```python
from build123d import *

# Parameters (mm, degrees)
F0_R     = 99.8962025771
F1_DEPTH = 50
F2_R     = 7.3881969702
F3_DEPTH = 50.001
F4_DEPTH = 50
F5_DEPTH = 20


with BuildPart() as f1:
    # F0 (on Front) → F1 (new body)
    with BuildSketch(Plane.XZ):
        Circle(F0_R)
    extrude(amount=F1_DEPTH)

    # F2 (on face) → F3 (cut, through all)
    with BuildSketch(Plane.XZ.offset(50)):
        Circle(F2_R)
    extrude(amount=-F3_DEPTH, mode=Mode.SUBTRACT)

    # F4 (add): a face of the model
    f4_faces = [f1.faces().sort_by_distance(p)[0] for p in [
        (-97.0707112869, -50, 0),
    ]]
    extrude(f4_faces, amount=F4_DEPTH)

    # F5 (cut): a face of the model
    f5_faces = [f1.faces().sort_by_distance(p)[0] for p in [
        (-97.0707112869, -100, 0),
    ]]
    extrude(f5_faces, amount=-F5_DEPTH, mode=Mode.SUBTRACT)


solid = f1.part
```
Can you work these out from the model? Positions are in its coordinate system, mm. Coordinates: 2 decimals unless noted, no trailing zeros. Order: outer loops, then holes, each group sorted by start corner. A loop starts at its lowest first (then second) coordinate and runs counter-clockwise, first axis right, second up.
1. I'm going to push flat-ended pins straight in: pin 1 (12 mm diameter, centred on x = 20, z = 35, fed in from +Y); pin 2 (3 mm diameter, centred on y = -32, z = -70.5, fed in from +X); pin 3 (10 mm diameter, centred on x = -9.5, y = -15, fed in from -Z); pin 4 (9 mm diameter, centred on x = 0, z = 0, fed in from -Y). Where does each tip first touch, or does it pass through?
2. If we section it at A-A (x = 0): Please give me the cut outline in (y, z), then the cut area to 3 significant figures.
3. If we section it at C-C (y = -18): Please give me the cut outline in (x, z), then the cut area to 3 significant figures.
4. I need wall thicknesses on line 1 (Z direction, x = 0, y = -72); line 2 (X direction, y = -33, z = 1); line 3 (Z direction, x = 62, y = -51). Which ranges of each line are inside material? Lowest first, please.
5. If we section it at B-B (z = 0): Please give me the cut outline in (x, y), then the cut area to 3 significant figures.
6. If we section it at D-D (x = -24.5): Please give me the cut outline in (y, z), then the cut area to 3 significant figures.
Entries:
1. pin 1: stops at y = 0
1. pin 2: stops at x = 72.24
1. pin 3: stops at z = -99.79
1. pin 4: passes through
2. outline: (-80, -99.9) - (0, -99.9) - (0, -7.39) - (-80, -7.39) - close; (-80, 7.39) - (0, 7.39) - (0, 99.9) - (-80, 99.9) - close
2. area: 14,800 mm2
3. outline: circle Ø199.79 at (0, 0); hole circle Ø14.78 at (0, 0)
3. area: 31,200 mm2
4. line 1: z = -99.9 to -7.39, 7.39 to 99.9
4. line 2: x = -99.89 to -7.32, 7.32 to 99.89
4. line 3: z = -78.33 to 78.33
5. outline: (-99.9, -80) - (-7.39, -80) - (-7.39, 0) - (-99.9, 0) - close; (7.39, -80) - (99.9, -80) - (99.9, 0) - (7.39, 0) - close
5. area: 14,800 mm2
6. outline: (-80, -96.85) - (0, -96.85) - (0, 96.85) - (-80, 96.85) - close
6. area: 15,500 mm2
